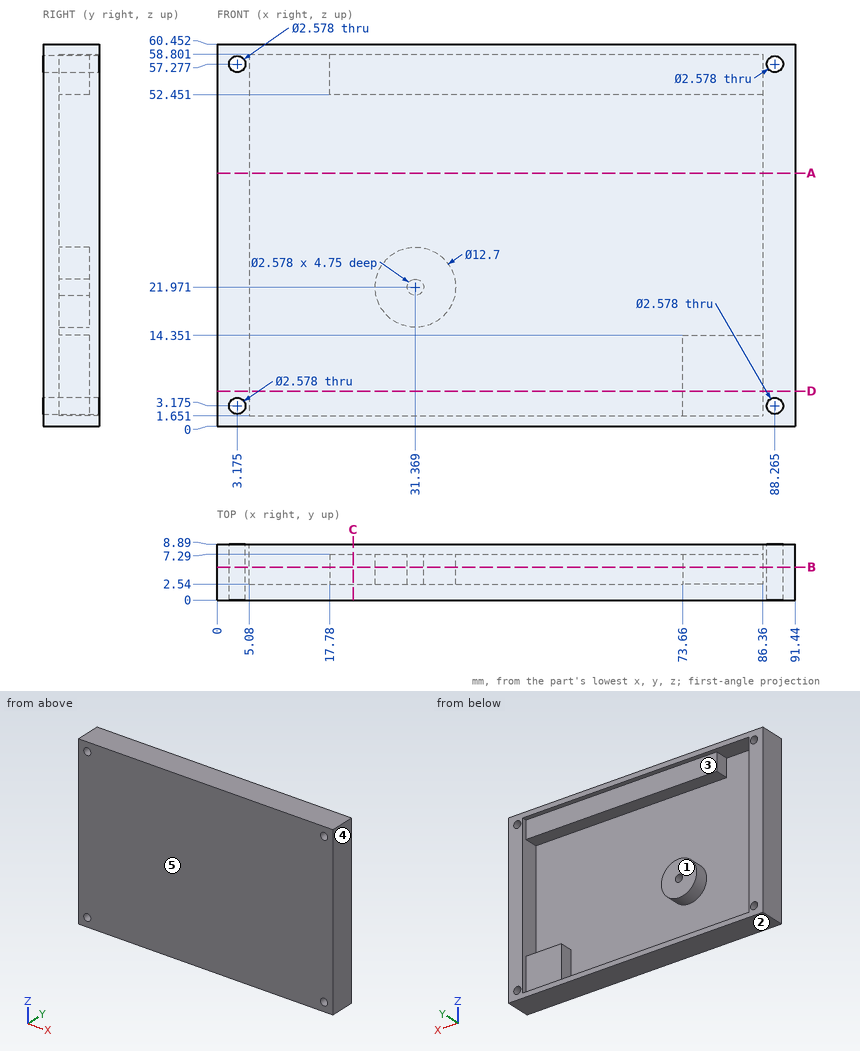
Here's the drawing with two shaded views (mm, measured from the low corner). I have some questions. A direction names the side the tool comes from. Give positions to 0.01 mm unless a question says otherwise; leave off trailing zeros. Loops run counter-clockwise (first coordinate to the right, second up) from the corner with the lowest first, then second, coordinate; pieces in that order, holes last. Notation, with made-up numbers: (-20, 42) -> (-10, 42) arc R15 ccw to (-10, 71) -> close; hole circle Ø5 at (22.5, 48). An arc over 180 degrees is marked (long way). One line per item, written item: value.
Q1. I'm going to push flat-ended pins straight in: pin 1 Ø0.8 at (x, z) = (31.5, 21.5) entering from +Y; pin 2 Ø10 at (x, z) = (33.5, 19) entering from +Y. Where does each tip first touch, or does it pass through?
Answers follow:
pin 1: y = 2.54
pin 2: y = 7.29
Q2. We'd pull the mould along X, two halves only. Please class the marked faces 3, 4 and 5: pulls with the +X half, pulls with the -X half, needs draft (parallel to the pull), parting line crosses it, or undercut.
Answers follow:
face 3: undercut
face 4: pulls with the +X half
face 5: needs draft
Q3. If I drill on line 1 along Z through (x, y) = (24.5, 3.5); line 2 along X through (y, z) = (3, 18.5); line 3 along Z through (x, y) = (27, 5.25), over which ranges is the centre line in solid material (lowest first)?
Answers follow:
line 1: 0 to 1.65, 52.45 to 60.45
line 2: 0 to 5.08, 26.05 to 36.69, 86.36 to 91.44
line 3: 0 to 1.65, 17.36 to 26.58, 52.45 to 60.45
Q4. Suppose I cut it at D-D on z = 5.5. Please give me the cut outline in (x, y), then the cut area to 3 significant figures.
Answers follow:
outline: (0, 0) -> (91.44, 0) -> (91.44, 8.89) -> (86.36, 8.89) -> (86.36, 7.29) -> (73.66, 7.29) -> (73.66, 2.54) -> (5.08, 2.54) -> (5.08, 8.89) -> (0, 8.89) -> close
area: 357 mm^2
Q5. On a 3-axis mill with a long thin cutter (end or side, diameter ignored), from which of +Z, -Z, +X, -X, +Y, -Y can I reach the whole of each face in a straight line? I mean the marked faces 1 and 2. Say none if no direction works.
Answers follow:
face 1: +Y
face 2: -Z, +X, -X, +Y, -Y
Q6. Suppose I cut it at B-B on y = 5.25. State how many separate pieces and enclosed holes the cut face has, then the cut area to 3 significant figures.
Answers follow:
separate pieces: 2
enclosed holes: 6
area: 1,580 mm^2
Q7. Suppose I cut it at C-C on x = 21.5. Please give me the cut outline in (y, z).
Answers follow:
outline: (0, 0) -> (8.89, 0) -> (8.89, 1.65) -> (2.54, 1.65) -> (2.54, 52.45) -> (7.29, 52.45) -> (7.29, 58.8) -> (8.89, 58.8) -> (8.89, 60.45) -> (0, 60.45) -> close
Q8. Suppose I cut it at A-A on z = 40. Please give me the cut outline in (x, y).
Answers follow:
outline: (0, 0) -> (91.44, 0) -> (91.44, 8.89) -> (86.36, 8.89) -> (86.36, 2.54) -> (5.08, 2.54) -> (5.08, 8.89) -> (0, 8.89) -> close
